from build123d import *

# Parameters (mm, degrees)
F2_DEPTH    = 5.8
F3_T1_DEPTH = 17.3214031257
F3_T3_DEPTH = 5.8
F5_DEPTH    = 8.901
F6_R        = 2


# Not quite as in the source:
# - a fillet or chamfer that OpenCascade refuses, or shapes differently, is made with other operations: its cross-section is extruded or revolved along the edge and cut away or added


with BuildPart() as f2:
    # F1 (on Top) → F2 (new body)
    with BuildSketch(Plane.XY):
        Polygon((-7.2977824063, -1.970131098), (-7.2977824063, 0), (-7.2977824063, 1.970131098), (-5.8, 3.25), (0, 3.25), (0, 4.45), (-6.2428722575, 4.45), (-8.4977824063, 2.523158448), (-8.4977824063, 0), (-8.4977824063, -2.523158448), (-6.2428722575, -4.45), (0, -4.45), (0, -3.25), (-5.8, -3.25), align=None)
    extrude(amount=F2_DEPTH)

    # F3: fillet of radius 5 on 4 edges, made by hand

    # F3_s2 → F3_t1 (cut)
    with BuildSketch(Plane.XY.offset(-5.7607015629)):
        with BuildLine():
            ThreePointArc((-6.7459644775, -4.0201030507), (-8.0387575415, -2.3116140275), (-8.4977824063, -0.2188778229))
            Line((-8.4977824063, -0.2188778229), (-8.5977824063, -0.2188778229))
            Line((-8.5977824063, -0.2188778229), (-8.5977824063, -2.5692440605))
            Line((-8.5977824063, -2.5692440605), (-6.8109281189, -4.0961275552))
            Line((-6.8109281189, -4.0961275552), (-6.7459644775, -4.0201030507))
        make_face()
        with BuildLine():
            ThreePointArc((-8.4977824063, 0.2188778229), (-8.0387575415, 2.3116140275), (-6.7459644775, 4.0201030507))
            Line((-6.7459644775, 4.0201030507), (-6.8109281189, 4.0961275552))
            Line((-6.8109281189, 4.0961275552), (-8.5977824063, 2.5692440605))
            Line((-8.5977824063, 2.5692440605), (-8.5977824063, 0.2188778229))
            Line((-8.5977824063, 0.2188778229), (-8.4977824063, 0.2188778229))
        make_face()
    extrude(amount=F3_T1_DEPTH, mode=Mode.SUBTRACT)

    # F3_s4 → F3_t3 (join)
    with BuildSketch(Plane.XY):
        with BuildLine():
            ThreePointArc((-7.2977824063, 0.3185391867), (-6.9081559253, -1.6165205064), (-5.8, -3.25))
            Line((-5.8, -3.25), (-5.8700443519, -3.3213707837))
            ThreePointArc((-5.8700443519, -3.3213707837), (-6.6138548446, -2.6860900535), (-7.3627460478, -2.0461556025))
            Line((-7.3627460478, -2.0461556025), (-7.3977824063, -1.970131098))
            Line((-7.3977824063, -1.970131098), (-7.3977824063, 0.3185391867))
            Line((-7.3977824063, 0.3185391867), (-7.2977824063, 0.3185391867))
        make_face()
        with BuildLine():
            ThreePointArc((-7.2977824063, -0.3185391867), (-6.9081559253, 1.6165205064), (-5.8, 3.25))
            Line((-5.8, 3.25), (-5.8700443519, 3.3213707837))
            ThreePointArc((-5.8700443519, 3.3213707837), (-6.6138548446, 2.6860900535), (-7.3627460478, 2.0461556025))
            Line((-7.3627460478, 2.0461556025), (-7.3977824063, 1.970131098))
            Line((-7.3977824063, 1.970131098), (-7.3977824063, -0.3185391867))
            Line((-7.3977824063, -0.3185391867), (-7.2977824063, -0.3185391867))
        make_face()
    extrude(amount=F3_T3_DEPTH)

    # F4 (on face) → F5 (cut, through all)
    with BuildSketch(Plane.XZ.offset(4.45)):
        with BuildLine():
            Line((-4.6214361287, 2.9), (-3.1214361287, 2.9))
            Line((-3.1214361287, 2.9), (-1.6214361287, 2.9))
            ThreePointArc((-1.6214361287, 2.9), (-3.1214361287, 4.4), (-4.6214361287, 2.9))
        make_face()
        with BuildLine():
            Line((-1.6214361287, 2.9), (-3.1214361287, 2.9))
            Line((-3.1214361287, 2.9), (-4.6214361287, 2.9))
            ThreePointArc((-4.6214361287, 2.9), (-3.1214361287, 1.4), (-1.6214361287, 2.9))
        make_face()
    extrude(amount=-F5_DEPTH, mode=Mode.SUBTRACT)

    # F6
    f6_edges = [f2.edges().sort_by_distance(p)[0] for p in [
        (0, 3.85, 5.8),
        (0, -3.85, 5.8),
        (0, 3.85, 0),
        (0, -3.85, 0),
    ]]
    fillet(f6_edges, radius=F6_R)


solid = f2.part
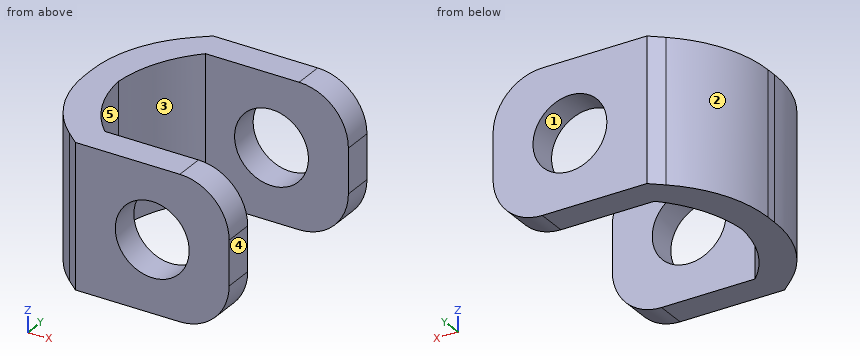
Could you check a few things on this model? Use its own coordinates, in mm. Face numbers are marked on the shaded views. A direction names the side the tool comes from. Round coordinates to 2 decimals unless told otherwise and drop trailing zeros. Order: outer loops, then holes, each group sorted by start corner. A loop starts at its lowest first (then second) coordinate and runs counter-clockwise, first axis right, second up.
Q1. Imagine slicing it at C-C, the plane x = -4. List the corners of the cut face in (y, z) for me.
Geometry says:
outline: (-4.45, 0) - (-3.25, 0) - (-3.25, 1.68) - (-4.45, 1.68) - close; (-4.45, 4.12) - (-3.25, 4.12) - (-3.25, 5.8) - (-4.45, 5.8) - close; (3.25, 0) - (4.45, 0) - (4.45, 1.68) - (3.25, 1.68) - close; (3.25, 4.12) - (4.45, 4.12) - (4.45, 5.8) - (3.25, 5.8) - close
Q2. Please list where these lines run through material, in increasing order: probe 1 along Y at (x, z) = (-0.5, 4); probe 2 along X at (y, z) = (4.05, 2.9); probe 3 along Y at (x, z) = (-6.75, 3.35).
Geometry says:
probe 1: y = -4.45 to -3.25, 3.25 to 4.45
probe 2: x = -6.71 to -4.62, -1.62 to 0
probe 3: y = -4.02 to -1.96, 1.96 to 4.02
Q3. Which directions (+Z, -Z, +X, -X, +Y, -Y) give clear straight access to the entire face, cutting with the end or side of a thin tool? Please do the marked faces 4 and 5.
Geometry says:
face 4: +Z, -Z, +X, +Y, -Y
face 5: +Z, -Z, +X
Q4. Thinking about a two-plate mould opening in Y: for the marked faces 1, 2 and 3, which applies, released by +Y, released by -Y, zero draft, split by the parting line, or undercut?
Geometry says:
face 1: zero draft
face 2: released by +Y
face 3: undercut
Q5. Imagine slicing it at A-A, the plane z = 2.9. List the corners of the cut face in (x, y) for me.
Geometry says:
outline: (-8.5, -0.22) arc R5 ccw to (-6.75, -4.02) - (-6.24, -4.45) - (-4.62, -4.45) - (-4.62, -3.25) - (-5.8, -3.25) arc R5 cw to (-7.29, 0) arc R5 cw to (-5.8, 3.25) - (-4.62, 3.25) - (-4.62, 4.45) - (-6.24, 4.45) - (-6.75, 4.02) arc R5 ccw to (-8.5, 0.22) - close; (-1.62, -4.45) - (0, -4.45) - (0, -3.25) - (-1.62, -3.25) - close; (-1.62, 3.25) - (0, 3.25) - (0, 4.45) - (-1.62, 4.45) - close
Q6. Imagine slicing it at B-B, the plane x = -1.25. List the corners of the cut face in (y, z) for me, then the cut area to 3 significant figures.
Geometry says:
outline: (-4.45, 0.15) - (-3.25, 0.15) - (-3.25, 5.65) - (-4.45, 5.65) - close; (3.25, 0.15) - (4.45, 0.15) - (4.45, 5.65) - (3.25, 5.65) - close
area: 13.2 mm2
Q7. Imagine slicing it at D-D, the plane z = 4. List the corners of the cut face in (x, y) for me.
Geometry says:
outline: (-8.5, -0.22) arc R5 ccw to (-6.75, -4.02) - (-6.24, -4.45) - (-4.14, -4.45) - (-4.14, -3.25) - (-5.8, -3.25) arc R5 cw to (-7.29, 0) arc R5 cw to (-5.8, 3.25) - (-4.14, 3.25) - (-4.14, 4.45) - (-6.24, 4.45) - (-6.75, 4.02) arc R5 ccw to (-8.5, 0.22) - close; (-2.1, -4.45) - (-0.01, -4.45) - (-0.01, -3.25) - (-2.1, -3.25) - close; (-2.1, 3.25) - (-0.01, 3.25) - (-0.01, 4.45) - (-2.1, 4.45) - close
